The model under review builds one solid part; all positions refer to its coordinate system, in mm. A direction names the side the tool comes from. Coordinates: 2 decimals unless noted, no trailing zeros. Write each loop counter-clockwise with the first axis right and the second up, starting at its lowest first coordinate (ties: lowest second). Pieces come first, ordered by that corner, then holes. Notation, with made-up numbers: (73.25, -30) - (126.25, -30) arc R18 cw to (126.25, -10) - close; hole circle Ø6 at (36, 15.25). An arc over 180 degrees is marked (long way). Use one line per item in the form item = value. Start each with the question number.
```python
from build123d import *

# Parameters (mm, degrees)
F1_DEPTH = 25.4


with BuildPart() as f1:
    # F0 (on Right) → F1 (new body)
    with BuildSketch(Plane.YZ):
        with BuildLine():
            ThreePointArc((0, 0), (12.7, 12.7), (25.4, 0))
            ThreePointArc((25.4, 0), (0, -25.4), (-25.4, 0))
            ThreePointArc((-25.4, 0), (-18.958987, 21.197135), (-1.813726, 35.227287))
            Line((-1.813726, 35.227287), (111.273858, 81.81964))
            ThreePointArc((111.273858, 81.81964), (182.712446, 140.278607), (209.55, 228.6))
            ThreePointArc((209.55, 228.6), (88.899999, 349.250003), (-31.75, 228.599999))
            ThreePointArc((-31.75, 228.599999), (50.800002, 146.050003), (133.35, 228.600003))
            ThreePointArc((133.35, 228.600003), (88.9, 273.050003), (44.45, 228.600003))
            Line((44.45, 228.600003), (50.8, 228.600003))
            ThreePointArc((50.8, 228.600003), (88.9, 266.700003), (127, 228.600003))
            ThreePointArc((127, 228.600003), (50.8, 152.400003), (-25.4, 228.600003))
            ThreePointArc((-25.4, 228.600003), (88.9, 342.900003), (203.2, 228.600003))
            ThreePointArc((203.2, 228.600003), (177.435949, 143.811464), (108.854904, 87.690855))
            Line((108.854904, 87.690855), (-4.23268, 41.098502))
            ThreePointArc((-4.23268, 41.098502), (-24.235486, 24.72999), (-31.75, -1e-06))
            ThreePointArc((-31.75, -1e-06), (0, -31.75), (31.75, -2e-06))
            ThreePointArc((31.75, -2e-06), (12.700001, 19.05), (-6.35, 0))
            Line((-6.35, 0), (0, 0))
        make_face()
    extrude(amount=F1_DEPTH)


solid = f1.part
```
1. Take a section at B-B (z = 200). State the section outline as (x, y) points, plus the area to 3 significant figures.
2. The part is to be moulded in two halves that separate along Z. For faces 1 (the cylindrical face through (12.522, 181.978, 139.192)), 2 (the cylindrical face through (12.52, 91.55, 349.22)), 3 (the flat face through (12.52, 53.94, 58.2)), 4 (the flat face through (25.4, 88, 160)), say which applies: released by +Z, released by -Z, zero draft, split by the parting line, or undercut.
3. For P1, Ø10, axis at x = 3, z = 123, coming from the -Y side; P2, Ø5, axis at x = 11.5, z = 128, coming from the +Y side; P3, Ø3, axis at x = 14, y = -4, coming from the -Z side, all flat-tipped, find the tip position at first contact; note any pin that passes through.
4. For L1, parallel to Z at x = 24, y = 73; L2, parallel to Z at x = 18.5, y = -7; L3, parallel to Y at x = 4.25, z = 230, list the stretches that pass through material, from the lowest coordinate up.
5. Take a section at A-A (y = 12.7). State the section outline as (x, z) points, plus the area to 3 significant figures.
6. Take a section at D-D (x = 5.5). State the section outline as (y, z) points, plus the area to 3 significant figures.
7. For faces 5 (the cylindrical face through (12.522, -0.698, -31.742)), 6 (the cylindrical face through (12.522, -24.03, 25.034)), 7 (the cylindrical face through (12.522, 86.387, 342.872)), list the 3-axis set-ups (+Z, -Z, +X, -X, +Y, -Y) from which the entire face can be reached by the end or side of a thin tool; tool diameter is ignored.
8. Take a section at C-C (y = 88.9). State the section outline as (x, z) points.
Returned:
q1.outline = (0, -26.64) - (25.4, -26.64) - (25.4, -19.83) - (0, -19.83) - close; (0, 121.43) - (25.4, 121.43) - (25.4, 128.24) - (0, 128.24) - close; (0, 200.49) - (25.4, 200.49) - (25.4, 206.95) - (0, 206.95) - close
q1.area = 510 mm²
q2.face_1 = released by -Z
q2.face_2 = released by +Z
q2.face_3 = undercut
q2.face_4 = zero draft
q3.P1 = 155.65
q3.P2 = 175.61
q3.P3 = -31.65
q4.L1 = 66.05 to 72.92, 149.09 to 155.71, 263.22 to 270.11, 341.79 to 348.2
q4.L2 = -30.97 to -24.42, 32.61 to 39.85, 169.66 to 178.95, 290.79 to 301.81
q4.L3 = -31.74 to -25.39, 44.47 to 50.83, 126.97 to 133.33, 203.19 to 209.54
q5.outline = (0, -29.1) - (25.4, -29.1) - (25.4, -22) - (0, -22) - close; (0, 12.7) - (25.4, 12.7) - (25.4, 19.05) - (0, 19.05) - close; (0, 41.21) - (25.4, 41.21) - (25.4, 48.07) - (0, 48.07) - close; (0, 155.37) - (25.4, 155.37) - (25.4, 162.61) - (0, 162.61) - close; (0, 313.79) - (25.4, 313.79) - (25.4, 322.14) - (0, 322.14) - close
q5.area = 912 mm²
q6.outline = (-31.75, 0) arc R31.75 ccw to (31.75, 0) arc R19.05 ccw to (-6.35, 0) - (0, 0) arc R12.7 cw to (25.4, 0) arc R25.4 cw to (-25.4, 0) arc R38.1 cw to (-1.81, 35.23) - (111.27, 81.82) arc R158.75 ccw to (209.55, 228.6) arc R120.65 ccw to (-31.75, 228.6) arc R82.55 ccw to (133.35, 228.6) arc R44.45 ccw to (44.45, 228.6) - (50.8, 228.6) arc R38.1 cw to (127, 228.6) arc R76.2 cw to (-25.4, 228.6) arc R114.3 cw to (203.2, 228.6) arc R152.4 cw to (108.85, 87.69) - (-4.23, 41.1) arc R44.45 ccw to start
q6.area = 7,890 mm²
q7.face_5 = -Z, +X, -X
q7.face_6 = +X, -X, -Y
q7.face_7 = +X, -X
q8.outline = (0, 72.6) - (25.4, 72.6) - (25.4, 79.47) - (0, 79.47) - close; (0, 155.37) - (25.4, 155.37) - (25.4, 162.61) - (0, 162.61) - close; (0, 266.7) - (25.4, 266.7) - (25.4, 273.05) - (0, 273.05) - close; (0, 342.9) - (25.4, 342.9) - (25.4, 349.25) - (0, 349.25) - close
